Print and shaded views of the part. All mm, measured from the part's lowest x, y and z. Coordinates: 2 decimals unless noted, no trailing zeros. Order: outer loops, then holes, each group sorted by start corner. A loop starts at its lowest first (then second) coordinate and runs counter-clockwise, first axis right, second up.
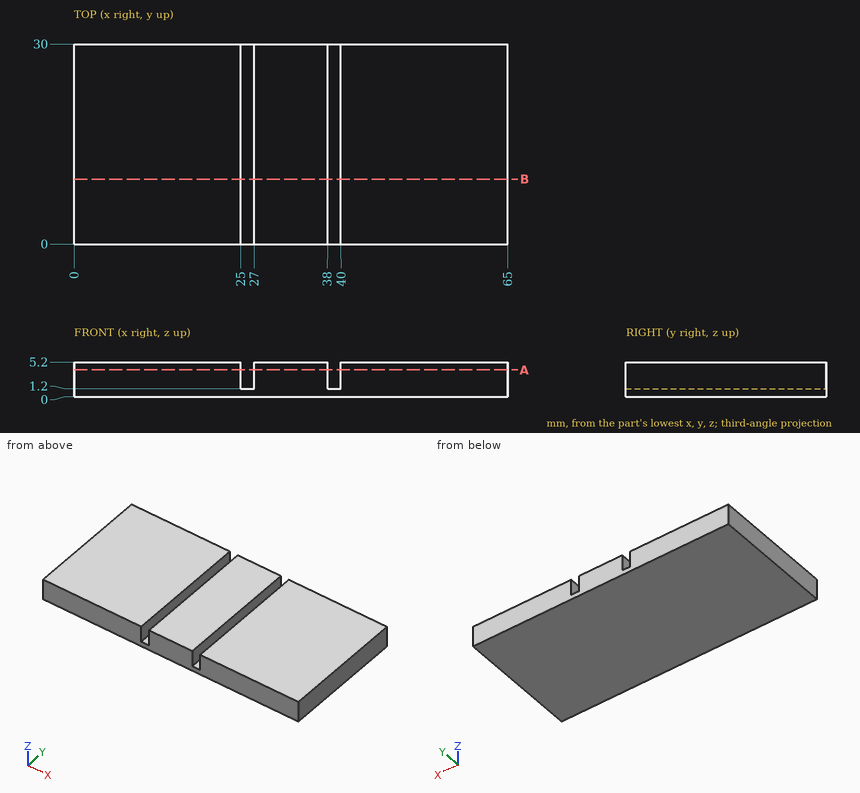
Q1. Drop a flat-ended pin along its axis: P1, Ø1, axis at x = 45, z = 2, coming from the -Y side. Give the stop position or say it passes through.
Established:
P1: stops at y = 0
Q2. Cut at B-B, the plane y = 9.75. List the corners of the cut face in (x, z), plus the area to 3 significant figures.
Established:
outline: (0, 0) - (65, 0) - (65, 5.2) - (40, 5.2) - (40, 1.2) - (38, 1.2) - (38, 5.2) - (27, 5.2) - (27, 1.2) - (25, 1.2) - (25, 5.2) - (0, 5.2) - close
area: 322 mm2
Q3. Probe line 1 (X direction, y = 29, z = 1.6); line 2 (Z direction, x = 38.5, y = 5). List the from-to ranges inside material, lowest first.
Established:
line 1: x = 0 to 25, 27 to 38, 40 to 65
line 2: z = 0 to 1.2
Q4. Cut at A-A, the plane z = 4.05. List the corners of the cut face in (x, y), plus the area to 3 significant figures.
Established:
outline: (0, 0) - (25, 0) - (25, 30) - (0, 30) - close; (27, 0) - (38, 0) - (38, 30) - (27, 30) - close; (40, 0) - (65, 0) - (65, 30) - (40, 30) - close
area: 1,830 mm2
